For this review, use the dimensioned drawing (mm, ordinates from the lowest corner) and the shaded views. A direction names the side the tool comes from. Give positions to 0.01 mm unless a question says otherwise; leave off trailing zeros. Order: outer loops, then holes, each group sorted by start corner. A loop starts at its lowest first (then second) coordinate and runs counter-clockwise, first axis right, second up. Notation, with made-up numbers: (18, 84) - (63, 84) arc R12 cw to (63, 95) - close; hole circle Ø3 at (28, 57.25). An arc over 180 degrees is marked (long way). Answer as CSV lines item,"result". Start each with the question number.
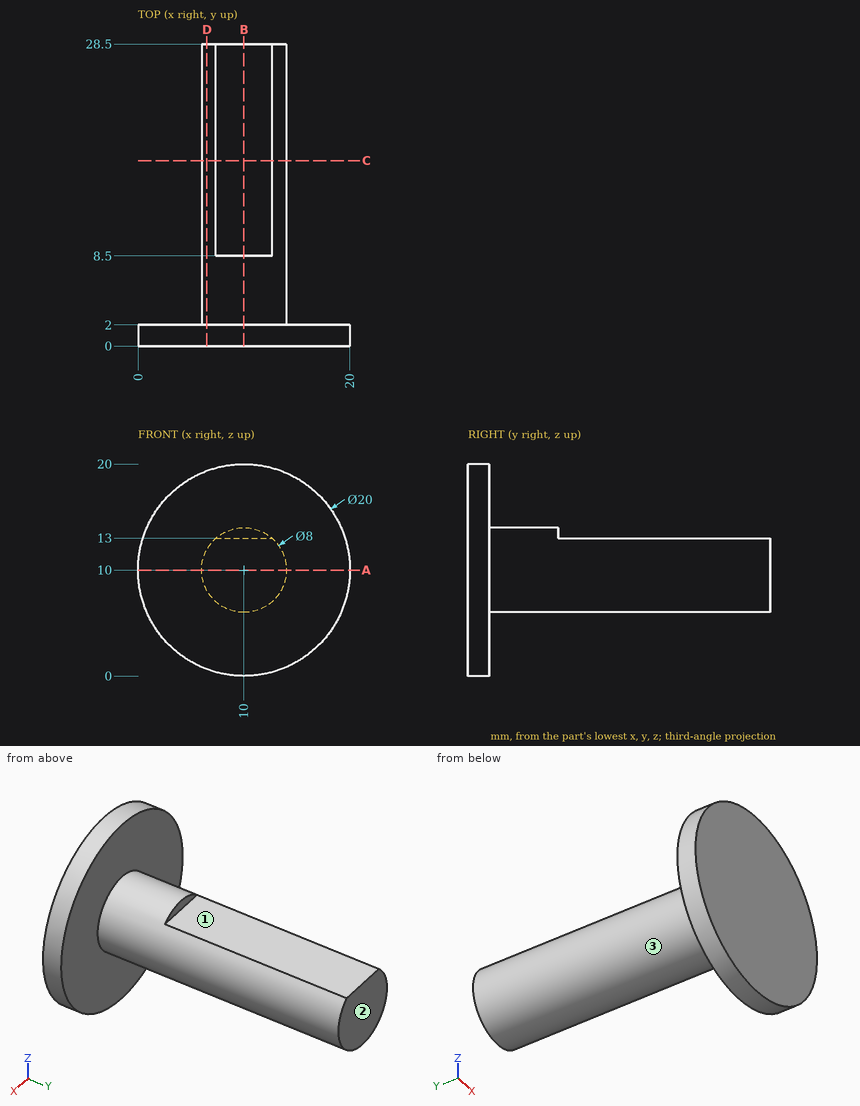
Item 1: For line 1 along Y through (x, z) = (18.5, 11.5); line 2 along X through (y, z) = (24.75, 9.75); line 3 along Z through (x, y) = (13, 3.25), list the stretches that pass through material, from the lowest coordinate up.
Item 2: Take a section at D-D on x = 6.5. Write out the cut boundary in (y, z), and give its area (3 significant figures).
Item 3: Take a section at B-B on x = 10. Write out the cut boundary in (y, z), and give its area (3 significant figures).
Item 4: Take a section at A-A on z = 10. Write out the cut boundary in (x, y).
Item 5: Take a section at C-C on y = 17.5. Write out the cut boundary in (x, z).
Item 6: Machinability: for the marked faces 1, 2 and 3, which of the approach directions +Z, -Z, +X, -X, +Y, -Y give a long, thin tool a straight path to every point of the face, cutting with its end or side? Answer none if there is none.
Item 7: Clearance check with flat-ended pins moving along their axes: pin 1 (1.5 mm diameter, centred on y = 20.5, z = 9.5, fed in from +X); pin 2 (10 mm diameter, centred on y = 8.5, z = 12, fed in from -X); pin 3 (1 mm diameter, centred on x = 14, y = 14.5, fed in from -Z). State where each tip first meets the part, or that it passes through.
Data:
1,line 1,"y = 0 to 2"
1,line 2,"x = 6.01 to 13.99"
1,line 3,"z = 7.35 to 12.65"
2,outline,"(0, 0.63) - (2, 0.63) - (2, 8.06) - (28.5, 8.06) - (28.5, 11.94) - (2, 11.94) - (2, 19.37) - (0, 19.37) - close"
2,area,"140 mm^2"
3,outline,"(0, 0) - (2, 0) - (2, 6) - (28.5, 6) - (28.5, 13) - (8.5, 13) - (8.5, 14) - (2, 14) - (2, 20) - (0, 20) - close"
3,area,"232 mm^2"
4,outline,"(0, 0) - (20, 0) - (20, 2) - (14, 2) - (14, 28.5) - (6, 28.5) - (6, 2) - (0, 2) - close"
5,outline,"(7.35, 13) arc R4 ccw (long way) to (12.65, 13) - close"
6,face 1,"+Z, +X, -X, +Y"
6,face 2,"+Z, -Z, +X, -X, +Y"
6,face 3,"+Y"
7,pin 1,"stops at x = 14"
7,pin 2,"stops at x = 6"
7,pin 3,"stops at z = 8.06"
